Source: CAD feature listing. Evaluate the final solid. Frame: model axes, mm. A direction names the side the tool comes from. Give positions to 0.01 mm unless a question says otherwise; leave off trailing zeros. Order: outer loops, then holes, each group sorted by start corner. A loop starts at its lowest first (then second) coordinate and runs counter-clockwise, first axis right, second up. Notation, with made-up numbers: (77.25, 24.5) - (101.25, 24.5) arc R15 cw to (101.25, 50.5) - close; hole circle Ø7 at (76, 18). An arc over 180 degrees is marked (long way). Write each question's results on one line, items separated by ' | '. Start each with the question number.
Item 1: Line query: line 1 along X through (y, z) = (8, 10.7); line 2 along Y through (x, z) = (25, 11.5); line 3 along Z through (x, y) = (-5.5, 8). Output: solid intervals per line, ascending.
Item 2: Set-up query: faces 4 (the cylindrical face through (9.41, 8.54, -8.99)), 5 (the flat face through (0, 6, 8)), 6 (the cylindrical face through (-9.41, 8.54, 8.99)), 7 (the flat face through (15, 6, -9)), 8 (the flat face through (0, 8, -10)). Return all of +Z, -Z, +X, -X, +Y, -Y with unobstructed straight access to the full face (end or side cutting, diameter ignored); none if empty.
Item 3: Section D-D on x = -0.5. Output: boundary loops of the cut face in (y, z), and give its area (3 significant figures).
Item 4: Section C-C on z = 9. Output: boundary loops of the cut face in (x, y).
Item 5: Contact query for flat-ended pins moving along their axis: pin 1 Ø1.6 at (x, z) = (5, -9) entering from +Y; pin 2 Ø1 at (x, y) = (7.5, 6.5) entering from +Z; pin 3 Ø2 at (y, z) = (4, -9.5) entering from -X. Output: stop coordinate, or through.
Item 6: Section A-A on x = 10. Output: boundary loops of the cut face in (y, z), and give its area (3 significant figures).
Item 7: Mould query, pull axis X, two halves, no side actions, for faces 1 (the flat face through (0, 8, 10)), 2 (the cylindrical face through (-18.085, 3.093, -10.955)), 3 (the flat face through (-17, 3, -10)). Classes: released by +X, released by -X, zero draft, split by the parting line, or undercut.
Item 8: Section B-B on y = 3.25. Output: boundary loops of the cut face in (x, z).
```python
from build123d import *
from build123d.topology import SkipClean

# Parameters (mm, degrees)
SKETCH_1_W               = 50
SKETCH_1_H               = 25
EXTRUDE_1_DEPTH          = 10
CUT_EXTRUDE_1_REACH      = 54.5
SKETCH_3_W               = 16
SKETCH_3_H               = 9
CUT_EXTRUDE_2_DEPTH      = 53.5
SKETCH_14_W              = 50
SKETCH_14_H              = 5
CUT_EXTRUDE_5_DEPTH      = 2.5
SKETCH_15_W              = 50
SKETCH_15_H              = 5
CUT_EXTRUDE_6_DEPTH      = 2.5
HOLE_WIZARD_M2_1_D       = 1.6
HOLE_WIZARD_M2_1_DEPTH   = 2
HOLE_WIZARD_M2_2_D       = 1.6
HOLE_WIZARD_M2_2_DEPTH   = 2
SKETCH_19_W              = 10
SKETCH_19_H              = 9
CUT_EXTRUDE_10_DEPTH     = 2
SKETCH_21_R              = 8
EXTRUDE_5_DEPTH          = 2.5
SKETCH_22_W              = 10
SKETCH_22_H              = 9
CUT_EXTRUDE_12_DEPTH     = 2
CUT_EXTRUDE_START        = -2.5
CUT_EXTRUDE_13_OUTLINE_R = 3
CUT_EXTRUDE_13_DEPTH     = 2.5
SKETCH_17_R              = 8.2
CUT_EXTRUDE_15_DEPTH     = 10
EXTRUDE_6_DEPTH          = 3
FILLET_1_R               = 1
FILLET_2_R               = 1


# Read off the part's stored shape, not the designer's step: 切除-拉伸13
with BuildPart() as part:
    # 草图1 → 凸台-拉伸1 (new body)
    with BuildSketch(Plane(origin=(0, 0, 0), x_dir=(1, 0, 0), z_dir=(0, 1, 0))):
        Rectangle(SKETCH_1_W, SKETCH_1_H)
    extrude(amount=EXTRUDE_1_DEPTH)

    # 草图2 → 切除-拉伸1 (cut, up to next)
    with BuildSketch(Plane(origin=(25, 0, 0), x_dir=(0, 0, -1), z_dir=(1, 0, 0)), mode=Mode.PRIVATE) as cut_extrude_1_sk1:
        with BuildLine():
            Line((-12.5, 0), (-7.5, 0))
            ThreePointArc((-7.5, 0), (-11.035533906, 1.464466094), (-12.5, 5))
            Line((-12.5, 5), (-12.5, 0))
        make_face()
    cut_extrude_1_tool1 = extrude(cut_extrude_1_sk1.sketch, amount=-CUT_EXTRUDE_1_REACH, mode=Mode.PRIVATE) & part.part
    # 草图2 → 切除-拉伸1 (cut, up to next)
    with BuildSketch(Plane(origin=(25, 0, 0), x_dir=(0, 0, -1), z_dir=(1, 0, 0)), mode=Mode.PRIVATE) as cut_extrude_1_sk2:
        with BuildLine():
            Line((12.5, 5), (12.5, 0))
            Line((12.5, 0), (7.5, 0))
            ThreePointArc((7.5, 0), (11.035533906, 1.464466094), (12.5, 5))
        make_face()
    cut_extrude_1_tool2 = extrude(cut_extrude_1_sk2.sketch, amount=-CUT_EXTRUDE_1_REACH, mode=Mode.PRIVATE) & part.part
    add(cut_extrude_1_tool1.solids().sort_by_distance((25, 1.11684, 11.38316))[0], mode=Mode.SUBTRACT)
    add(cut_extrude_1_tool2.solids().sort_by_distance((25, 1.11684, -11.38316))[0], mode=Mode.SUBTRACT)

    # 草图3 → 切除-拉伸2 (cut, through all)
    with BuildSketch(Plane(origin=(25, 0, 0), x_dir=(0, 0, -1), z_dir=(1, 0, 0))):
        with Locations((0, 5.5)):
            Rectangle(SKETCH_3_W, SKETCH_3_H)
    extrude(amount=-CUT_EXTRUDE_2_DEPTH, mode=Mode.SUBTRACT)

    # 草图14 → 切除-拉伸5 (cut)
    with BuildSketch(Plane(origin=(0, 0, -12.5), x_dir=(-1, 0, 0), z_dir=(0, 0, -1))):
        with Locations((0, 7.5)):
            Rectangle(SKETCH_14_W, SKETCH_14_H)
    extrude(amount=-CUT_EXTRUDE_5_DEPTH, mode=Mode.SUBTRACT)

    # 草图15 → 切除-拉伸6 (cut)
    with BuildSketch(Plane.XY.offset(12.5)):
        with Locations((0, 7.5)):
            Rectangle(SKETCH_15_W, SKETCH_15_H)
    extrude(amount=-CUT_EXTRUDE_6_DEPTH, mode=Mode.SUBTRACT)

    # M2 螺纹孔1
    with Locations(Plane(origin=(0, 0, -10), x_dir=(-1, 0, 0), z_dir=(0, 0, -1))):
        with Locations((-10, 8)):
            Hole(HOLE_WIZARD_M2_1_D / 2, depth=HOLE_WIZARD_M2_1_DEPTH)

    # M2 螺纹孔2
    with Locations(Plane.XY.offset(10)):
        with Locations((-10, 8)):
            Hole(HOLE_WIZARD_M2_2_D / 2, depth=HOLE_WIZARD_M2_2_DEPTH)

    # 草图19 → 切除-拉伸10 (cut)
    with BuildSketch(Plane.XY.offset(-8)):
        with Locations((-20, 5.5)):
            Rectangle(SKETCH_19_W, SKETCH_19_H)
        with Locations((20, 5.5)):
            Rectangle(SKETCH_19_W, SKETCH_19_H)
    extrude(amount=-CUT_EXTRUDE_10_DEPTH, mode=Mode.SUBTRACT)

    # 草图21 → 凸台-拉伸5 (add)
    with SkipClean():  # the faces are left unmerged after this step: merging them gives an invalid solid
        with BuildSketch(Plane.XY.offset(10)):
            with Locations((25, 8)):
                Circle(SKETCH_21_R)
            with Locations((-25, 8)):
                Circle(SKETCH_21_R)
        extrude(amount=EXTRUDE_5_DEPTH)

    # 草图22 → 切除-拉伸12 (cut)
    with SkipClean():  # the faces are left unmerged after this step: merging them gives an invalid solid
        with BuildSketch(Plane.XY.offset(10)):
            with Locations((-20, 5.5)):
                Rectangle(SKETCH_22_W, SKETCH_22_H)
            with Locations((20, 5.5)):
                Rectangle(SKETCH_22_W, SKETCH_22_H)
        extrude(amount=-CUT_EXTRUDE_12_DEPTH, mode=Mode.SUBTRACT)

    # 切除-拉伸13 outline → 切除-拉伸13 (cut)
    with SkipClean():  # the faces are left unmerged after this step: merging them gives an invalid solid
        with BuildSketch(Plane.XY.offset(12.5).offset(CUT_EXTRUDE_START)):
            with Locations((25, 8)):
                Circle(CUT_EXTRUDE_13_OUTLINE_R)
            with Locations((-25, 8)):
                Circle(CUT_EXTRUDE_13_OUTLINE_R)
        extrude(amount=CUT_EXTRUDE_13_DEPTH, mode=Mode.SUBTRACT)

    # 草图17 → 切除-拉伸15 (cut)
    with SkipClean():  # the faces are left unmerged after this step: merging them gives an invalid solid
        with BuildSketch(Plane(origin=(0, 0, -10), x_dir=(-1, 0, 0), z_dir=(0, 0, -1))):
            with Locations((-25, 7.5)):
                Circle(SKETCH_17_R)
            with Locations((25, 7.5)):
                Circle(SKETCH_17_R)
        extrude(amount=CUT_EXTRUDE_15_DEPTH, mode=Mode.SUBTRACT)

    # 草图24 → 凸台-拉伸6 (add)
    with SkipClean():  # the faces are left unmerged after this step: merging them gives an invalid solid
        with BuildSketch(Plane.ZY.offset(25)):
            with BuildLine():
                Line((10, 1), (-10, 1))
                Line((-10, 1), (-10, 0.669872981))
                ThreePointArc((-10, 0.669872981), (-8.794095226, 0.170370869), (-7.5, 0))
                Line((-7.5, 0), (7.5, 0))
                ThreePointArc((7.5, 0), (8.794095226, 0.170370869), (10, 0.669872981))
                Line((10, 0.669872981), (10, 1))
            make_face()
        extrude(amount=EXTRUDE_6_DEPTH)

    # 圆角1
    # the kernel refuses this fillet: 1 mm, written as the material it adds along each edge
    with BuildSketch(Plane(origin=(15, 1, 8), x_dir=(0, 0, -1), z_dir=(-1, 0, 0))) as fillet_1_piece_1:
        with BuildLine():
            CenterArc((FILLET_1_R, -FILLET_1_R), FILLET_1_R, 90, 90)
            Line((0, -FILLET_1_R), (0, 0))
            Line((0, 0), (FILLET_1_R, 0))
        make_face()
    extrude(amount=30)
    with BuildSketch(Plane(origin=(15, 1, -8), x_dir=(0, 0, 1), z_dir=(-1, 0, 0))) as fillet_1_piece_2:
        with BuildLine():
            CenterArc((FILLET_1_R, FILLET_1_R), FILLET_1_R, 180, 90)
            Line((0, FILLET_1_R), (0, 0))
            Line((0, 0), (FILLET_1_R, 0))
        make_face()
    extrude(amount=30)

    # 圆角2
    fillet_2_edges = [part.edges().sort_by_distance(p)[0] for p in [
        (0, 5, -10),
        (0, 5, 10),
    ]]
    fillet(fillet_2_edges, radius=FILLET_2_R)


solid = part.part
```
Evaluation:
1) line 1: x = -33 to -28, -22 to -17, 17 to 22, 28 to 33 | line 2: y = 0 to 5, 11 to 16 | line 3: z = -10 to -8, 8 to 10
2) face 4: -Z | face 5: +X, -X, +Y | face 6: +Z | face 7: +X, +Y | face 8: -Z, +X, -X, +Y
3) outline: (0, -7.5) arc R5 ccw to (5, -12.5) - (5, -11) arc R1 cw to (6, -10) - (10, -10) - (10, -8) - (2, -8) arc R1 cw to (1, -7) - (1, 7) arc R1 cw to (2, 8) - (10, 8) - (10, 10) - (6, 10) arc R1 cw to (5, 11) - (5, 12.5) arc R5 ccw to (0, 7.5) - close | area: 71.1 mm^2
4) outline: (-28, 0.23) - (25, 0.23) - (25, 1) - (15, 1) - (15, 10) - (-15, 10) - (-15, 1) - (-28, 1) - close; hole circle Ø1.6 at (-10, 8)
5) pin 1: stops at y = 10 | pin 2: stops at z = 10 | pin 3: stops at x = -18.06
6) outline: (0, -7.5) arc R5 ccw to (5, -12.5) - (5, -11) arc R1 cw to (6, -10) - (7.2, -10) - (7.2, -8) - (2, -8) arc R1 cw to (1, -7) - (1, 7) arc R1 cw to (2, 8) - (10, 8) - (10, 10) - (6, 10) arc R1 cw to (5, 11) - (5, 12.5) arc R5 ccw to (0, 7.5) - close; (8.8, -10) - (10, -10) - (10, -8) - (8.8, -8) - close | area: 67.9 mm^2
7) face 1: undercut | face 2: released by -X | face 3: zero draft
8) outline: (-31.44, 10) - (-15, 10) - (-15, 8) - (15, 8) - (15, 10) - (31.44, 10) - (31.44, 12.5) - (18.56, 12.5) - (18.56, 12.18) - (-18.56, 12.18) - (-18.56, 12.5) - (-31.44, 12.5) - close; (-17.99, -12.18) - (17.99, -12.18) - (17.99, -10) - (15, -10) - (15, -8) - (-15, -8) - (-15, -10) - (-17.99, -10) - close
